Check sheet for the modelled part. Datum: model origin and axes. Units: mm. Round coordinates to 2 decimals unless told otherwise and drop trailing zeros. Write each loop counter-clockwise with the first axis right and the second up, starting at its lowest first coordinate (ties: lowest second). Pieces come first, ordered by that corner, then holes. Notation, with made-up numbers: M 12.5,50.5 L 33.5,50.5 A33 cw 33.5,86.5 Z; hole C -12,-13.75 d7. An arc over 180 degrees is marked long. One line per item, written item: value.
Autodesk Inventor part; units mm, degrees
ref_plane "YZ Plane" through (0, 0, 0) normal (1, 0, 0) x (0, 1, 0)
ref_plane "XZ Plane" through (0, 0, 0) normal (0, 1, 0) x (-1, 0, 0)
ref_plane "XY Plane" through (0, 0, 0) normal (0, 0, 1) x (1, 0, 0)
sketch "Sketch1" plane through (0, 0, 0) normal (0, 1, 0) x (-1, 0, 0)
  line L0 (0, 0) -> (215.9, 0)
  line L1 (215.9, 0) -> (215.9, -215.9)
  line L2 (215.9, -215.9) -> (0, -215.9)
  line L3 (0, -215.9) -> (0, 0)
  dimension "d0" = 215.9
  dimension "d1" = 215.9
extrude "Extrusion1" add sketch "Sketch1" along normal blind 3.175
sketch "Sketch2" plane through (0, 3.175, 0) normal (0, 1, 0) x (1, 0, 0)
  line L0 (-291.9068, 6.35) -> (0, 6.35)
  line L1 (0, 6.35) -> (0, 293.5185)
  line L2 (0, 293.5185) -> (-291.9068, 293.5185)
  line L3 (-291.9068, 293.5185) -> (-291.9068, 6.35)
  line L4 (-215.9, 0) -> (0, 0)
  line L5 (0, 0) -> (0, 215.9)
  point P0 (-26, 79.35)
  point P1 (-79, 31.35)
  point P2 (-79, 186.35)
  point P3 (-26, 144.35)
  dimension "d4" = 138
  dimension "d5" = 26
  dimension "d6" = 79
  dimension "d7" = 25
  dimension "d8" = 79
  dimension "d9" = 26
  dimension "d10" = 73
  dimension "d11" = 180
  dimension "d12" = 6.35
  dimension "d13" = 0
hole "Hole1" at (-26, 3.175, -79.35) at (-79, 3.175, -31.35) at (-79, 3.175, -186.35) at (-26, 3.175, -144.35) direction (0, -1, 0) diameter 6 end through all
properties part number "side panel v1.2"
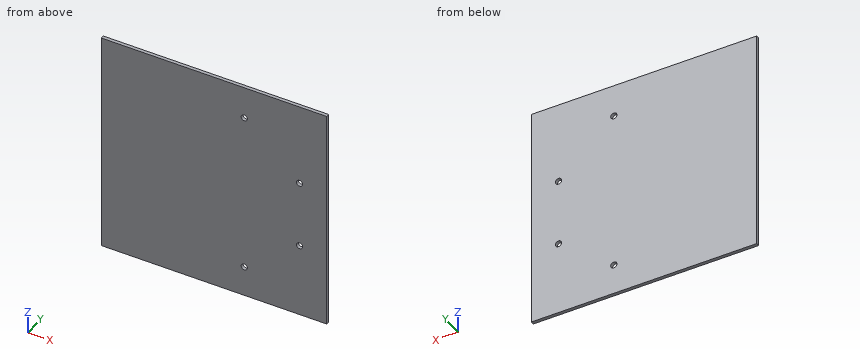
Q1. Sectioned sample at B-B on z = -186.35. Enter the section's corners in (x, y) (3 decimals).
Completed:
outline: M -215.9,0 L -82,0 L -82,3.175 L -215.9,3.175 Z; M -76,0 L 0,0 L 0,3.175 L -76,3.175 Z
Q2. Depth check by flat-ended pin: P1, Ø5.5, axis at x = -26, z = -79.35, coming from the -Y side. Enter the tip coordinate at first touch or a pass-through.
Completed:
P1: through
Q3. Sectioned sample at C-C on x = -79. Enter the section's corners in (y, z) (3 decimals), and give its area (3 significant figures).
Completed:
outline: M 0,-215.9 L 3.175,-215.9 L 3.175,-189.35 L 0,-189.35 Z; M 0,-183.35 L 3.175,-183.35 L 3.175,-34.35 L 0,-34.35 Z; M 0,-28.35 L 3.175,-28.35 L 3.175,0 L 0,0 Z
area: 647 mm^2
Q4. Sectioned sample at A-A on x = -26. Enter the section's corners in (y, z) (3 decimals), and give its area (3 significant figures).
Completed:
outline: M 0,-215.9 L 3.175,-215.9 L 3.175,-147.35 L 0,-147.35 Z; M 0,-141.35 L 3.175,-141.35 L 3.175,-82.35 L 0,-82.35 Z; M 0,-76.35 L 3.175,-76.35 L 3.175,0 L 0,0 Z
area: 647 mm^2
Q5. Scan lines: line 1 (Z direction, x = -26, y = 1.1); line 2 (X direction, y = 1.65, z = -144.35); line 3 (X direction, y = 1.2, z = -31.35). Record each from-to range of solid material in increasing order. Write a range as [from, to].
Completed:
line 1: [-215.9, -147.35], [-141.35, -82.35], [-76.35, 0]
line 2: [-215.9, -29], [-23, 0]
line 3: [-215.9, -82], [-76, 0]
Q6. Sectioned sample at D-D on z = -79.35. Enter the section's corners in (x, y) (3 decimals).
Completed:
outline: M -215.9,0 L -29,0 L -29,3.175 L -215.9,3.175 Z; M -23,0 L 0,0 L 0,3.175 L -23,3.175 Z
